from build123d import *

# Parameters (mm, degrees)
SKETCH1_W  = 78
SKETCH1_H  = 78
COIL_DEPTH = 7


with BuildPart() as part:
    # Sketch1 → Coil (new body)
    with BuildSketch(Plane(origin=(0, 0, 0), x_dir=(1, 0, 0), z_dir=(0, 1, 0))):
        with BuildLine():
            Line((0.2, -11), (81.8, -11))
            ThreePointArc((81.8, -11), (81.941421356, -10.941421356), (82, -10.8))
            Line((82, -10.8), (82, 70.8))
            ThreePointArc((82, 70.8), (81.941421356, 70.941421356), (81.8, 71))
            Line((81.8, 71), (0.2, 71))
            ThreePointArc((0.2, 71), (0.058578644, 70.941421356), (0, 70.8))
            Line((0, 70.8), (0, -10.8))
            ThreePointArc((0, -10.8), (0.058578644, -10.941421356), (0.2, -11))
        make_face()
        with Locations((41, 30)):
            Rectangle(SKETCH1_W, SKETCH1_H, mode=Mode.SUBTRACT)
    extrude(amount=COIL_DEPTH)


solid = part.part
The model under review builds one solid part; all positions refer to its coordinate system, in mm. A direction names the side the tool comes from. Round coordinates to 2 decimals unless told otherwise and drop trailing zeros. Order: outer loops, then holes, each group sorted by start corner. A loop starts at its lowest first (then second) coordinate and runs counter-clockwise, first axis right, second up. Notation, with made-up numbers: (23, 8) - (58, 8) arc R22 ccw to (58, 19) - close; hole circle Ø7 at (-31.75, 56.25). An arc over 180 degrees is marked (long way). Use one line per item in the form item = value.
Q1. Add section A-A on z = -14.5. Give the boundary of the cut face in (x, y), then the cut area to 3 significant figures.
Response values:
outline = (0, 0) - (2, 0) - (2, 7) - (0, 7) - close; (80, 0) - (82, 0) - (82, 7) - (80, 7) - close
area = 28.0 mm^2
Q2. Mouldability with a two-part tool opening along Z and no side actions: class faces 3 (the flat face through (40, 3, 9)), 4 (the flat face through (40, 3, 11)), 5 (the flat face through (2, 3, -29)), 6 (the flat face through (82, 3, -29)) as pulls with the +Z half, pulls with the -Z half, needs draft (parallel to the pull), parting line crosses it, or undercut.
Response values:
face_3 = undercut
face_4 = pulls with the +Z half
face_5 = undercut
face_6 = needs draft
Q3. Tool access review of faces 1 (the flat face through (42, 3, -71)), 2 (the flat face through (80, 3, -29)): name each direction out of +Z, -Z, +X, -X, +Y, -Y from which nothing blocks a thin tool from reaching the whole face with its end or side.
Response values:
face_1 = -Z, +X, -X, +Y, -Y
face_2 = +Y, -Y
Q4. To check wall thickness, follow line 1 (X direction, y = 1.75, z = 1.5); line 2 (Z direction, x = 21.5, y = 3.5). State the ranges of each line that lie inside material, in increasing order.
Response values:
line_1 = 0 to 2, 80 to 82
line_2 = -71 to -69, 9 to 11
Q5. Add section C-C on y = 1.75. Give the boundary of the cut face in (x, z), then the cut area to 3 significant figures.
Response values:
outline = (0, -70.8) arc R0.2 ccw to (0.2, -71) - (81.8, -71) arc R0.2 ccw to (82, -70.8) - (82, 10.8) arc R0.2 ccw to (81.8, 11) - (0.2, 11) arc R0.2 ccw to (0, 10.8) - close; hole (2, -69) - (80, -69) - (80, 9) - (2, 9) - close
area = 640 mm^2
Q6. Add section B-B on x = 73. Give the boundary of the cut face in (y, z).
Response values:
outline = (0, -71) - (7, -71) - (7, -69) - (0, -69) - close; (0, 9) - (7, 9) - (7, 11) - (0, 11) - close
